Could you check a few things on this model? Use its own coordinates, in mm. A direction names the side the tool comes from. Give positions to 0.01 mm unless a question says otherwise; leave off trailing zeros. Order: outer loops, then holes, each group sorted by start corner. A loop starts at its lowest first (then second) coordinate and runs counter-clockwise, first axis right, second up.
from build123d import *

# Parameters (mm, degrees)
SKETCH1_R                = 43.3
BOSS_EXTRUDE1_DEPTH      = 0.58
BOSS_EXTRUDE2_START      = -0.58
SKETCH2_R                = 36.83
BOSS_EXTRUDE2_DEPTH      = 65
BOSS_EXTRUDE3_DEPTH      = 1.34
BOSS_EXTRUDE3_DEPTH_BACK = 1.34
SKETCH3_W                = 20.2
SKETCH3_H                = 90.8
SKETCH3_R                = 1.95
BOSS_EXTRUDE4_START      = 64.42
SKETCH4_R                = 37.849999992
BOSS_EXTRUDE4_DEPTH      = 2.15
BOSS_EXTRUDE5_START      = 36.703
SKETCH4_2_R              = 37.849999992
BOSS_EXTRUDE5_DEPTH      = 2.15
BOSS_EXTRUDE6_START      = -65
SKETCH5_R                = 14.299999975
BOSS_EXTRUDE6_DEPTH      = 85.4
BOSS_EXTRUDE7_DEPTH      = 50.8
FILLET1_R                = 8.89
BOSS_EXTRUDE8_START      = -65
SKETCH6_R                = 38.227
BOSS_EXTRUDE8_DEPTH      = 12.954


with BuildPart() as part:
    # Sketch1 → Boss-Extrude1 (new body)
    with BuildSketch(Plane(origin=(0, 0, 0), x_dir=(0, 0, -1), z_dir=(1, 0, 0))):
        Circle(SKETCH1_R)
    extrude(amount=BOSS_EXTRUDE1_DEPTH)

    # Sketch2 → Boss-Extrude2 (add)
    with BuildSketch(Plane(origin=(0.58, 0, 0), x_dir=(0, 0, -1), z_dir=(1, 0, 0)).offset(BOSS_EXTRUDE2_START)):
        Circle(SKETCH2_R)
    extrude(amount=BOSS_EXTRUDE2_DEPTH)

    # Sketch3 → Boss-Extrude3 (add, two sides: drawn at the far end of the back side and taken through both)
    with BuildSketch(Plane.XY.offset(-BOSS_EXTRUDE3_DEPTH_BACK)):
        with Locations((36.25, 0)):
            Rectangle(SKETCH3_W, SKETCH3_H)
        with Locations((36.25, 41.115)):
            Circle(SKETCH3_R, mode=Mode.SUBTRACT)
        with Locations((36.25, -41.115)):
            Circle(SKETCH3_R, mode=Mode.SUBTRACT)
    extrude(amount=BOSS_EXTRUDE3_DEPTH + BOSS_EXTRUDE3_DEPTH_BACK)

    # Sketch4 → Boss-Extrude4 (add)
    with BuildSketch(Plane(origin=(0.58, 0, 0), x_dir=(0, 0, -1), z_dir=(1, 0, 0)).offset(BOSS_EXTRUDE4_START)):
        Circle(SKETCH4_R)
    extrude(amount=-BOSS_EXTRUDE4_DEPTH)

    # Sketch4<2> → Boss-Extrude5 (add)
    with BuildSketch(Plane(origin=(0.58, 0, 0), x_dir=(0, 0, -1), z_dir=(1, 0, 0)).offset(BOSS_EXTRUDE5_START)):
        Circle(SKETCH4_2_R)
    extrude(amount=-BOSS_EXTRUDE5_DEPTH)

    # Sketch5 → Boss-Extrude6 (add)
    with BuildSketch(Plane(origin=(65, 0, 0), x_dir=(0, 0, -1), z_dir=(1, 0, 0)).offset(BOSS_EXTRUDE6_START)):
        with Locations(Location((0, 0, 0), (0, 0, 180))):
            Circle(SKETCH5_R)
    extrude(amount=BOSS_EXTRUDE6_DEPTH)

    # Sketch3<3> → Boss-Extrude7 (add)
    with BuildSketch(Plane.XY):
        with BuildLine():
            Line((40.850706358, 3.5), (46.850706358, 3.5))
            ThreePointArc((46.850706358, 3.5), (50.350706358, 0), (46.850706358, -3.5))
            Line((46.850706358, -3.5), (40.850706358, -3.5))
            ThreePointArc((40.850706358, -3.5), (37.350706358, 0), (40.850706358, 3.5))
        make_face()
    extrude(amount=BOSS_EXTRUDE7_DEPTH)

    # Fillet1
    # the kernel refuses this fillet: 8.89 mm, written as the material it adds along each edge
    with BuildSketch(Plane(origin=(0.58, 0, 0), x_dir=(0, 0, -1), z_dir=(0, 1, 0))) as fillet1_piece_1:
        with BuildLine():
            CenterArc((45.72, -8.554279631), FILLET1_R, 105.796172805, 74.203827195)
            Line((36.83, -8.554279631), (36.6522, -8.554279631))
            Line((36.6522, -8.554279631), (36.6522, 0))
            Line((36.6522, 0), (36.83, 0.1778))
            ThreePointArc((36.83, 0.1778), (40.065, 0.1778), (43.2516, 0.171085593))
            Line((43.2516, 0.171085593), (43.3, 0))
        make_face()
    revolve(axis=Axis((0.58, 0, 0), (-1, 0, 0)))

    # Sketch6 → Boss-Extrude8 (add)
    with BuildSketch(Plane(origin=(65, 0, 0), x_dir=(0, 0, -1), z_dir=(1, 0, 0)).offset(BOSS_EXTRUDE8_START)):
        Circle(SKETCH6_R)
    extrude(amount=BOSS_EXTRUDE8_DEPTH)


solid = part.part
Item 1: For pin 1 (4.5 mm diameter, centred on x = 31.5, y = -40, fed in from +Z); pin 2 (10 mm diameter, centred on x = 56.5, z = 6.5, fed in from -Y); pin 3 (2 mm diameter, centred on x = 67.5, z = 12, fed in from -Y), each with a flat end and sliding along its axis, tell me the tip position at first contact or that it passes through.
Findings:
pin 1: stops at z = 1.34
pin 2: stops at y = -36.8
pin 3: stops at y = -9.14
Item 2: Please list where these lines run through material, in increasing order: line 1 along Y through (x, z) = (36.25, -0.55) (3 decimals); line 2 along X through (y, z) = (-13.5, -34.5); line 3 along Y through (x, z) = (36, 0).
Findings:
line 1: y = -45.4 to -43.065, -39.165 to 39.165, 43.065 to 45.4
line 2: x = 0 to 12.95, 35.13 to 37.28, 62.85 to 65
line 3: y = -45.4 to -43.05, -39.18 to 39.18, 43.05 to 45.4
Item 3: We'd pull the mould along X, two halves only. Please class faces 1 (the flat face through (37.283, 3, 37)), 2 (the flat face through (62.85, -36.3, -8.2)), 3 (the flat face through (36, 45.4, 0)), 4 (the flat face through (85.4, 0, 0)): +X half, -X half, draft (parallel to the pull), parting line (faces both ways), or undercut.
Findings:
face 1: undercut
face 2: undercut
face 3: draft
face 4: +X half
Item 4: Imagine slicing it at A-A on z = 0. Give the number of separate pieces and of enclosed holes in the cut face, then the cut area to 3 significant figures.
Findings:
separate pieces: 1
enclosed holes: 2
area: 5,750 mm2
Item 5: For faces 5 (the flat face through (12.954, 31.3, 20)), 6 (the flat face through (37.283, 0, -37)), 7 (the flat face through (26.15, 41, 0)), 8 (the flat face through (26.15, -41, 0)), 9 (the cylindrical face through (75.06, -4.3, 13.64)), which set-ups out of +Z, -Z, +X, -X, +Y, -Y let a thin tool reach every point of the face, with its end or its side?
Findings:
face 5: none
face 6: -Z
face 7: +Z, -Z, +Y
face 8: +Z, -Z, -Y
face 9: +X
Item 6: Imagine slicing it at D-D on x = 6. List the corners of the cut face in (y, z) for me.
Findings:
outline: circle Ø76.45 at (0, 0)
